```python
from build123d import *

# Parameters (mm, degrees)
F0_R     = 50.1
F0_R_2   = 4.5
F1_DEPTH = 3
F2_R     = 12.5
F2_R_2   = 4.5
F3_DEPTH = 25


# Not quite as in the source:
# - a fillet or chamfer that OpenCascade refuses, or shapes differently, is made with other operations: its cross-section is extruded or revolved along the edge and cut away or added


with BuildPart() as f1:
    # F0 (on Front) → F1 (new body)
    with BuildSketch(Plane.XZ):
        Circle(F0_R)
        Circle(F0_R_2, mode=Mode.SUBTRACT)
    extrude(amount=F1_DEPTH)

    # F2 (on face) → F3 (join)
    with BuildSketch(Plane.XZ.offset(3)):
        Circle(F2_R)
        Circle(F2_R_2, mode=Mode.SUBTRACT)
    extrude(amount=F3_DEPTH)

    # F4: fillet of radius 5 on 2 edges, made by hand

    # F4_s1 → F4_t2 (revolve, cut)
    with BuildSketch(Plane.XY):
        with BuildLine():
            ThreePointArc((50.1, -3), (48.2560370926, -0.8166998673), (45.517424305, 0))
            Line((45.517424305, 0), (50.1, 0))
            Line((50.1, 0), (50.1, -3))
        make_face()
    revolve(axis=Axis((0, 0, 0), (0, -1, 0)), mode=Mode.SUBTRACT)

    # F4_s3 → F4_t4 (revolve, cut)
    with BuildSketch(Plane.XY):
        with BuildLine():
            ThreePointArc((4.5, -5), (5.9644660941, -1.4644660941), (9.5, 0))
            Line((9.5, 0), (4.5, 0))
            Line((4.5, 0), (4.5, -5))
        make_face()
    revolve(axis=Axis((0, 0, 0), (0, -1, 0)), mode=Mode.SUBTRACT)


solid = f1.part
```
Here's how the part is built. I have some questions about the finished solid (model axes, mm). A direction names the side the tool comes from. Coordinates: 2 decimals unless noted, no trailing zeros. Order: outer loops, then holes, each group sorted by start corner. A loop starts at its lowest first (then second) coordinate and runs counter-clockwise, first axis right, second up.
1) Imagine slicing it at A-A on z = 0. List the corners of the cut face in (x, y) for me, and give its area (3 significant figures).
2) Will these pins go through, and if not, where does the flat tip stop? pin 1 (5 mm diameter, centred on x = -17, y = -15.5, fed in from -Z); pin 2 (6 mm diameter, centred on y = -21.5, z = 9, fed in from -X); pin 3 (12 mm diameter, centred on x = -15.5, y = -18.5, fed in from +Z); pin 4 (12 mm diameter, centred on x = 9.5, y = -22.5, fed in from -Z).
3) Imagine slicing it at C-C on y = -14. List the corners of the cut face in (x, z) for me.
4) Which directions (+Z, -Z, +X, -X, +Y, -Y) give clear straight access to the entire face, cutting with the end or side of a thin tool? Please do faces 1 (the face through (0, -28, -5)), 2 (the face through (10, -3, -10)).
5) We'd pull the mould along X, two halves only. Please class faces 3 (the face through (-1, 0, 11)), 4 (the face through (11.923, -15.325, 3.755)), 5 (the face through (-0.59, -16.34, 4.46)): +X half, -X half, draft (parallel to the pull), parting line (faces both ways), or undercut.
6) Imagine slicing it at B-B on x = 0. List the corners of the cut face in (y, z) for me.
7) I need wall thicknesses on line 1 (Z direction, x = 0, y = -10.25); line 2 (Y direction, x = 10, z = 18.5); line 3 (X direction, y = -22.25, z = -4). Which ranges of each line are inside material? Lowest first, please.
Response values:
1. outline: (-50.1, -3) - (-12.5, -3) - (-12.5, -28) - (-4.5, -28) - (-4.5, -5) arc R5 ccw to (-9.5, 0) - (-45.52, 0) arc R5 ccw to start; (4.5, -28) - (12.5, -28) - (12.5, -3) - (50.1, -3) arc R5 ccw to (45.52, 0) - (9.5, 0) arc R5 ccw to (4.5, -5) - close
1. area: 655 mm2
2. pin 1: passes through
2. pin 2: stops at x = -10.97
2. pin 3: stops at z = 8.12
2. pin 4: stops at z = -12
3. outline: circle Ø25 at (0, 0); hole circle Ø9 at (0, 0)
4. face 1: +Z, -Z, +X, -X, -Y
4. face 2: -Y
5. face 3: draft
5. face 4: parting line
5. face 5: undercut
6. outline: (-28, -12.5) - (-3, -12.5) - (-3, -50.1) arc R5 ccw to (0, -45.52) - (0, -9.5) arc R5 ccw to (-5, -4.5) - (-28, -4.5) - close; (-28, 4.5) - (-5, 4.5) arc R5 ccw to (0, 9.5) - (0, 45.52) arc R5 ccw to (-3, 50.1) - (-3, 12.5) - (-28, 12.5) - close
7. line 1: z = -12.5 to -4.5, 4.5 to 12.5
7. line 2: y = -3 to 0
7. line 3: x = -11.84 to -2.06, 2.06 to 11.84
